```python
from build123d import *

# Parameters (mm, degrees)
SKETCH1_W                    = 320
SKETCH1_H                    = 12.5
CHAMFER1_SIZE                = 1.6
M10_TAPPED_HOLE1_D           = 8.5
M10_TAPPED_HOLE1_DEPTH       = 24.5
M10_TAPPED_HOLE1_CBORE_D     = 10
M10_TAPPED_HOLE1_CBORE_DEPTH = 20
M10_TAPPED_HOLE1_TIP         = 2.553657631


with BuildPart() as part:
    # Sketch1 → Revolve1 (revolve)
    with BuildSketch(Plane.XY, mode=Mode.PRIVATE) as revolve1_sk:
        with Locations((-160, 6.25)):
            Rectangle(SKETCH1_W, SKETCH1_H)
    revolve(revolve1_sk.sketch.rotate(Axis((0, 0, 0), (-1, 0, 0)), 90), axis=Axis((0, 0, 0), (-1, 0, 0)))

    # Chamfer1
    chamfer1_edges = [part.edges().sort_by_distance(p)[0] for p in [
        (-320, 0, 12.5),
        (0, 0, 12.5),
    ]]
    chamfer(chamfer1_edges, length=CHAMFER1_SIZE)

    # M10 Tapped Hole1
    with Locations(Plane.ZY.offset(320)):
        with Locations((0, 0)):
            CounterBoreHole(M10_TAPPED_HOLE1_D / 2, M10_TAPPED_HOLE1_CBORE_D / 2, M10_TAPPED_HOLE1_CBORE_DEPTH, depth=M10_TAPPED_HOLE1_DEPTH)
            with Locations((0, 0, -(M10_TAPPED_HOLE1_DEPTH + M10_TAPPED_HOLE1_TIP / 2))):  # 118° drill point
                Cone(0, M10_TAPPED_HOLE1_D / 2, M10_TAPPED_HOLE1_TIP, mode=Mode.SUBTRACT)


solid = part.part
```
Geometry: final body of the model. Coordinates: model frame, mm. A direction names the side the tool comes from. Round coordinates to 2 decimals unless told otherwise and drop trailing zeros. Order: outer loops, then holes, each group sorted by start corner. A loop starts at its lowest first (then second) coordinate and runs counter-clockwise, first axis right, second up. Notation, with made-up numbers: (60, -26.75) -> (117, -26.75) arc R34 cw to (117, 5.25) -> close; hole circle Ø10 at (74.25, -35.5). An arc over 180 degrees is marked (long way). Use CSV: the item, a comma, the result in double quotes. Start each with the question number.
1) First-contact query: pin 1 Ø12 at (x, z) = (-35, 3) entering from +Y; pin 2 Ø5 at (x, y) = (-257.5, 6) entering from -Z; pin 3 Ø1.5 at (x, z) = (-261.5, 2) entering from +Y; pin 4 Ø3 at (y, z) = (-1, 1.5) entering from -X. Flat tips, straight axial feed; report the tip coordinate or a pass-through.
2) Set-up query: faces 5 (the face through (-297.718, 3.584, -2.285)), 6 (the face through (-320, 5, 2)). Return all of +Z, -Z, +X, -X, +Y, -Y with unobstructed straight access to the full face (end or side cutting, diameter ignored); none if empty.
3) Material intervals for line 1 along Y through (x, z) = (-312.25, 0); line 2 along Y through (x, z) = (-23.5, 0); line 3 along X through (y, z) = (-6.25, 10.5), sorted ascending. Write a range as from..to.
4) Section A-A (x = -128). Return the cut outline in (y, z).
5) Draft query along Z for faces 1 (the face through (-300, -4, -2)), 2 (the face through (-157.782, -3.755, -11.923)), 3 (the face through (0, 0, 0)), 4 (the face through (-293.39, -0.72, -0.16)). Return one class per face: +Z half, -Z half, draft (parallel to the pull), parting line (faces both ways), or undercut.
Returned:
1,pin 1,"stops at y = 12.5"
1,pin 2,"stops at z = -12"
1,pin 3,"stops at y = 12.44"
1,pin 4,"stops at x = -294.93"
2,face 5,"-X"
2,face 6,"+Z, -Z, -X, +Y, -Y"
3,line 1,"y = -12.5..-5, 5..12.5"
3,line 2,"y = -12.5..12.5"
3,line 3,"x = -318.68..-1.32"
4,outline,"circle Ø25 at (0, 0)"
5,face 1,"undercut"
5,face 2,"parting line"
5,face 3,"draft"
5,face 4,"undercut"
